Autodesk Inventor part; units mm, degrees
ref_plane "YZ Plane" through (0, 0, 0) normal (1, 0, 0) x (0, 1, 0)
ref_plane "XZ Plane" through (0, 0, 0) normal (0, 1, 0) x (-1, 0, 0)
ref_plane "XY Plane" through (0, 0, 0) normal (0, 0, 1) x (1, 0, 0)
sketch "Sketch1" plane through (0, 0, 0) normal (1, 0, 0) x (0, 1, 0)
  circle A0 centre (-9.7574, -19.7073) radius 1.55 construction
  circle A1 centre (0, 0) radius 1.55 construction
  circle A2 centre (-9.7574, -19.7073) radius 2.55
  circle A3 centre (0, 0) radius 2.55
  line L0 (-6.0684, -24.2876) -> (12.7398, 12.1607) construction
  arc A4 (-12.2239, -24.4871) -> (-4.9776, -22.1738) centre (-9.7574, -19.7073) ccw
  circle A5 centre (0, 0) radius 5.7448
  line L1 (-4.9776, -22.1738) -> (5.1052, -2.6344)
  arc A6 (-4.9776, -22.1738) -> (-12.2239, -24.4871) centre (-9.7574, -19.7073) ccw
  line L2 (-14.5372, -17.2408) -> (-5.1904, 2.4623)
  line L3 (0, 0) -> (0, -27.0135) construction
  line L4 (0, 0) -> (-9.7574, -19.7073) construction
  point P0 (-10.1101, -25.5779)
  dimension "d0" = 5.1
  dimension "d1" = 5.1
  dimension "d3" = 11.4897
  dimension "d4" = 5.3787
  dimension "d5" = 21.8076
  dimension "d6" = 21.9875
extrude "Extrusion1" add sketch "Sketch1" along normal blind 4
sketch "Sketch2" plane through (4, 0, 0) normal (1, 0, 0) x (0, 0, -1)
  arc A0 (17.2408, -14.5372) -> (22.1738, -4.9776) centre (19.7073, -9.7574) ccw
  line L0 (22.1738, -4.9776) -> (2.6344, 5.1052)
  arc A1 (2.6344, 5.1052) -> (-2.4623, -5.1904) centre (0, 0) ccw
  line L1 (-2.4623, -5.1904) -> (17.2408, -14.5372) construction
  circle A2 centre (19.7073, -9.7574) radius 2.55 construction
  circle A3 centre (0, 0) radius 2.55 construction
  circle A4 centre (19.7073, -9.7574) radius 2.55 construction
  line L2 (-0.0042, 0.0021) -> (19.7073, -9.7574) construction
  circle A5 centre (17.8404, 11.2524) radius 1
  circle A6 centre (17.8404, 11.2524) radius 4
  line L3 (15.9937, 14.8006) -> (-2.6523, 5.0959)
  arc A7 (2.6344, 5.1052) -> (-2.4623, -5.1904) centre (0, 0) ccw
  line L4 (21.793, 11.8661) -> (25.0223, -8.9322)
  line L5 (-11.8641, -11.015) -> (9.5186, 32.1722)
  dimension "d11" = 2
  dimension "d12" = 8
  dimension "d18" = 16.7401
  dimension "d19" = 18
extrude "Extrusion2" add sketch "Sketch2" against normal up to surface (4 mm away)
sketch "Sketch3" plane through (4, 0, 0) normal (1, 0, 0) x (0, 0, -1)
  circle A0 centre (17.8404, 11.2524) radius 1
  circle A1 centre (17.8404, 11.2524) radius 2.5
  point P0 (0, 0)
  dimension "d15" = 5
extrude "Extrusion3" cut sketch "Sketch3" against normal blind 2
properties part number "Kauri modular camera mount mini" material "Brass, Soft Yellow"
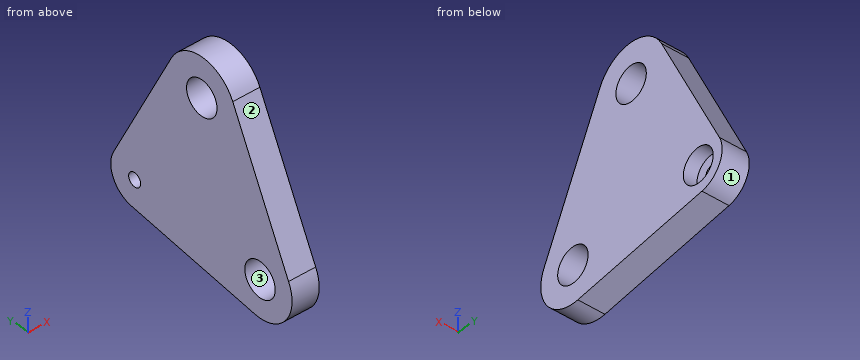
The model under review builds one solid part; all positions refer to its coordinate system, in mm. Face numbers are marked on the shaded views. Coordinates: 2 decimals unless noted, no trailing zeros. Write each loop counter-clockwise with the first axis right and the second up, starting at its lowest first coordinate (ties: lowest second). Pieces come first, ordered by that corner, then holes. Notation, with made-up numbers: M -2.5,36.25 L 51.5,36.25 A32 cw 51.5,66.25 Z; hole C 65,23 d3. An arc over 180 degrees is marked long. Put each result on its own line as item: value.
1) Add section D-D on z = -9.5. Give the boundary of the cut face in (x, y), then the cut area to 3 significant figures.
Computed:
outline: M 0,-10.87 L 4,-10.87 L 4,11.42 L 0,11.42 Z
area: 89.1 mm2
2) Add section B-B on x = 1.2. Give the boundary of the cut face in (y, z).
Computed:
outline: M -14.54,-17.24 A5.38 ccw -8.93,-25.02 L 11.87,-21.79 A4 ccw 14.8,-15.99 L 5.1,2.65 A5.74 ccw -5.19,2.46 Z; hole C -9.76,-19.71 d5.1; hole C 0,0 d5.1; hole C 11.25,-17.84 d2
3) Add section A-A on y = 0. Give the boundary of the cut face in (x, z), then the cut area to 3 significant figures.
Computed:
outline: M 0,-23.64 L 4,-23.64 L 4,-2.55 L 0,-2.55 Z; M 0,2.55 L 4,2.55 L 4,5.74 L 0,5.74 Z
area: 97.1 mm2
4) Add section C-C on z = 1.5. Give the boundary of the cut face in (x, y).
Computed:
outline: M 0,-5.65 L 4,-5.65 L 4,-2.06 L 0,-2.06 Z; M 0,2.06 L 4,2.06 L 4,5.7 L 0,5.7 Z
5) Draft analysis for pull direction Z (two halves, no side actions). For the marked faces 1, 2 and 3, state which applies: released by +Z, released by -Z, zero draft, split by the parting line, or undercut.
Computed:
face 1: split by the parting line
face 2: released by +Z
face 3: undercut
6) Clearance check with a flat-ended pin moving along its axis: pin 1 Ø2 at (x, y) = (2.5, -6) entering from +Z. State where the tip first meets the part, or that it passes through.
Computed:
pin 1: stops at z = 2.83
7) Wall thickness on probe 1 along Z at (x, y) = (3.5, 1); probe 2 along Z at (x, y) = (0.4, -10); probe 3 along Y at (x, z) = (0.8, -17.5): over which ranges is each line inside the solid? List them lowest first. Write a range as [from, to].
Computed:
probe 1: z = [-23.48, -2.35], [2.35, 5.66]
probe 2: z = [-25.08, -22.25], [-17.17, -7.68]
probe 3: y = [-14.66, -11.03], [-8.48, 10.31], [12.19, 15.24]
